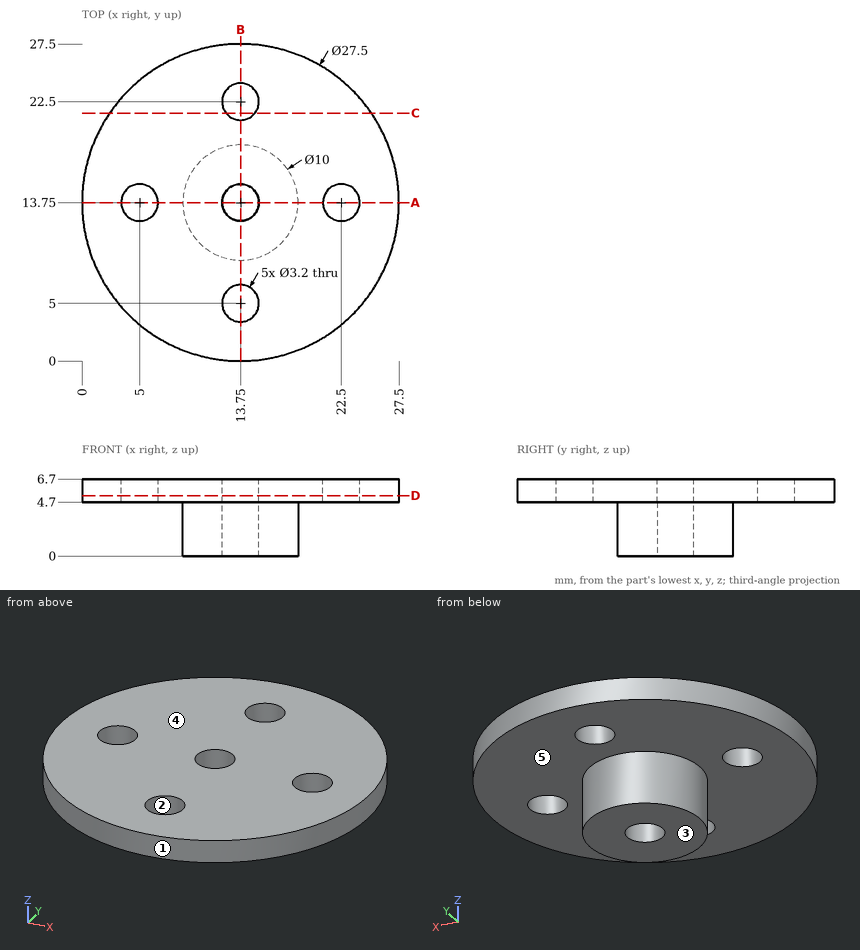
Can you work these out from the drawing? Everything is in mm from the part's minimum corner. A direction names the side the tool comes from. Round coordinates to 2 decimals unless told otherwise and drop trailing zeros. Order: outer loops, then holes, each group sorted by start corner. A loop starts at its lowest first (then second) coordinate and runs counter-clockwise, first axis right, second up. Notation, with made-up numbers: (-8.75, 46.5) - (21.25, 46.5) arc R28 ccw to (21.25, 78.5) - close; hole circle Ø6 at (6.25, 32). An arc over 180 degrees is marked (long way). Answer in a Markdown table with one row per item.
(1) Please list where these lines run through material, in increasing order: L1, parallel to Y at x = 13.75, z = 6.2; L2, parallel to Y at x = 13.75, z = 4.25; L3, parallel to X at y = 12.5, z = 5. Write a range as from..to.
From the geometry:
| item | result |
|---|---|
| L1 | y = 0..3.4, 6.6..12.15, 15.35..20.9, 24.1..27.5 |
| L2 | y = 8.75..12.15, 15.35..18.75 |
| L3 | x = 0.06..4, 6..12.75, 14.75..21.5, 23.5..27.44 |
(2) Suppose I cut it at A-A, the plane y = 13.75. Please give me the cut outline in (x, z), plus the area to 3 significant figures.
From the geometry:
| item | result |
|---|---|
| outline | (0, 4.7) - (3.4, 4.7) - (3.4, 6.7) - (0, 6.7) - close; (6.6, 4.7) - (8.75, 4.7) - (8.75, 0) - (12.15, 0) - (12.15, 6.7) - (6.6, 6.7) - close; (15.35, 0) - (18.75, 0) - (18.75, 4.7) - (20.9, 4.7) - (20.9, 6.7) - (15.35, 6.7) - close; (24.1, 4.7) - (27.5, 4.7) - (27.5, 6.7) - (24.1, 6.7) - close |
| area | 67.8 mm2 |
(3) Suppose I cut it at C-C, the plane y = 21.5. Please give me the cut outline in (x, z), plus the area to 3 significant figures.
From the geometry:
| item | result |
|---|---|
| outline | (2.39, 4.7) - (12.5, 4.7) - (12.5, 6.7) - (2.39, 6.7) - close; (15, 4.7) - (25.11, 4.7) - (25.11, 6.7) - (15, 6.7) - close |
| area | 40.4 mm2 |
(4) Suppose I cut it at D-D, the plane z = 5.25. Please give me the cut outline in (x, y).
From the geometry:
| item | result |
|---|---|
| outline | circle Ø27.5 at (13.75, 13.75); hole circle Ø3.2 at (5, 13.75); hole circle Ø3.2 at (13.75, 5); hole circle Ø3.2 at (13.75, 13.75); hole circle Ø3.2 at (13.75, 22.5); hole circle Ø3.2 at (22.5, 13.75) |
(5) Which directions (+Z, -Z, +X, -X, +Y, -Y) give clear straight access to the entire face, cutting with the end or side of a thin tool? Please do the marked faces 4 and 5.
From the geometry:
| item | result |
|---|---|
| face 4 | +Z, +X, -X, +Y, -Y |
| face 5 | -Z |
(6) For P1, Ø1.9, axis at x = 22.5, y = 13.75, coming from the -Z side; P2, Ø4, axis at y = 7.5, z = 5.5, coming from the -X side; P3, Ø1.5, axis at x = 22.5, z = 5.5, coming from the -Y side; P4, Ø4, axis at x = 24, z = 4.5, coming from the +Y side, each with a flat end and sliding along its axis, tell me the tip position at first contact or that it passes through.
From the geometry:
| item | result |
|---|---|
| P1 | passes through |
| P2 | stops at x = 0.67 |
| P3 | stops at y = 2.57 |
| P4 | stops at y = 24.74 |
(7) If we mould it in two halves opening along X, with no side actions, what happens to the marked faces 1, 2 and 3? For each: released by +X, released by -X, zero draft, split by the parting line, or undercut.
From the geometry:
| item | result |
|---|---|
| face 1 | split by the parting line |
| face 2 | undercut |
| face 3 | zero draft |
